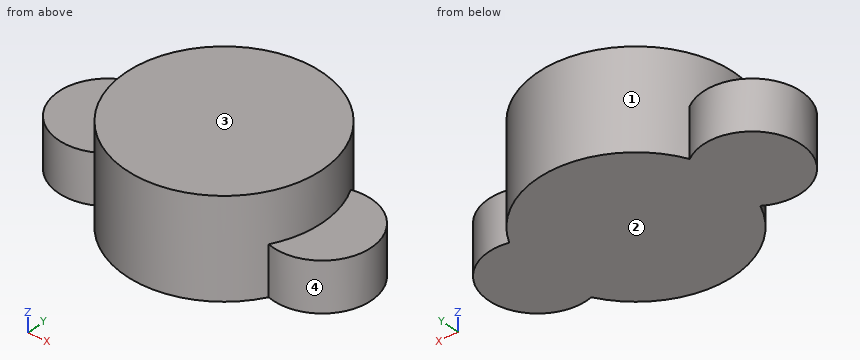
from build123d import *

# Parameters (mm, degrees)
F0_R     = 50
F1_DEPTH = 50
F2_R     = 25
F3_DEPTH = 25


with BuildPart() as f1:
    # F0 (on Top) → F1 (new body)
    with BuildSketch(Plane.XY):
        Circle(F0_R)
    extrude(amount=F1_DEPTH)

    # F2 (on Top) → F3 (join)
    with BuildSketch(Plane.XY):
        with Locations((50.145525, 0)):
            Circle(F2_R)
        with Locations((-59.403446, 0)):
            Circle(F2_R)
    extrude(amount=F3_DEPTH)


solid = f1.part
Design review of the part built by this model. Coordinates are the model's own, in mm. Face numbers are marked on the shaded views. A direction names the side the tool comes from. Give positions to 0.01 mm unless a question says otherwise; leave off trailing zeros. Loops run counter-clockwise (first coordinate to the right, second up) from the corner with the lowest first, then second, coordinate; pieces in that order, holes last. Notation, with made-up numbers: (-25, 40.5) -> (-10, 40.5) arc R22 cw to (-10, 75.5) -> close; hole circle Ø6 at (69, 12.5). An arc over 180 degrees is marked (long way). One line per question, with ' | ' between items. Start each with the question number.
(1) For line 1 (Y direction, x = 51, z = 3); line 2 (Z direction, x = -65.5, y = -4.5); line 3 (Y direction, x = -36, z = 31.5), list the stretches that pass through material, from the lowest coordinate up.
(2) We need section A-A (y = 0). State the section outline as (x, z) points.
(3) We need section C-C (x = 31). State the section outline as (y, z) points, and give its area (3 significant figures).
(4) Draft analysis for pull direction X (two halves, no side actions). For the marked faces 3 and 4, state which applies: +X half, -X half, draft (parallel to the pull), parting line (faces both ways), or undercut.
(5) We need section B-B (z = 29.5). State the section outline as (x, y) points.
(6) For the marked faces 1 and 2, list the 3-axis set-ups (+Z, -Z, +X, -X, +Y, -Y) from which the entire face can be reached by the end or side of a thin tool; tool diameter is ignored.
(7) Insertion check: P1, Ø1.5, axis at y = -26, z = 17.5, coming from the +X side; P2, Ø4, axis at x = 14.5, z = 14.5, coming from the +Y side; P3, Ø19.5, axis at x = -63, y = -0.5, coming from the +Z side. Each pin has a flat end and moves straight along its axis. Give the tip position at first contact, or say it passes through.
(8) We need section D-D (y = -11.5). State the section outline as (x, z) points.
The answers:
1) line 1: y = -24.99 to 24.99 | line 2: z = 0 to 25 | line 3: y = -34.7 to 34.7
2) outline: (-84.4, 0) -> (75.15, 0) -> (75.15, 25) -> (50, 25) -> (50, 50) -> (-50, 50) -> (-50, 25) -> (-84.4, 25) -> close
3) outline: (-39.23, 0) -> (39.23, 0) -> (39.23, 50) -> (-39.23, 50) -> close | area: 3,920 mm^2
4) face 3: draft | face 4: undercut
5) outline: circle Ø100 at (0, 0)
6) face 1: +Z | face 2: -Z, +X, -X, +Y, -Y
7) P1: stops at x = 43.16 | P2: stops at y = 48.41 | P3: stops at z = 25
8) outline: (-81.6, 0) -> (72.34, 0) -> (72.34, 25) -> (48.66, 25) -> (48.66, 50) -> (-48.66, 50) -> (-48.66, 25) -> (-81.6, 25) -> close
